Read the model definition and answer for the solid it produces. Units are mm, in the model's axes. A direction names the side the tool comes from. Coordinates: 2 decimals unless noted, no trailing zeros. Loops run counter-clockwise (first coordinate to the right, second up) from the corner with the lowest first, then second, coordinate; pieces in that order, holes last.
from build123d import *

# Parameters (mm, degrees)
SKETCH_1_W          = 21
SKETCH_1_H          = 31
EXTRUDE_1_DEPTH     = 20
CUT_EXTRUDE_5_REACH = 50.177
SKETCH_14_R         = 1.5
CUT_EXTRUDE_6_REACH = 50.177
SKETCH_15_R         = 1.5
EXTRUDE_2_DEPTH     = 1
EXTRUDE_START       = 1
EXTRUDE_3_DEPTH     = 1
SKETCH_4_R          = 1.5
CUT_EXTRUDE_1_DEPTH = 3
SKETCH_5_R          = 5
CUT_EXTRUDE_2_DEPTH = 4
SKETCH_6_W          = 9
SKETCH_6_H          = 29
EXTRUDE_START_2     = -8
SKETCH_7_R          = 1.5
EXTRUDE_4_DEPTH     = 8
EXTRUDE_START_3     = 20
SKETCH_8_R          = 5
EXTRUDE_5_DEPTH     = 20
SKETCH_10_R         = 1.75
CUT_EXTRUDE_4_DEPTH = 20
SKETCH_9_R          = 5
SKETCH_9_R_2        = 4
CUT_EXTRUDE_3_DEPTH = 1
SKETCH_11_R         = 2.85
EXTRUDE_6_DEPTH     = 3.5
FILLET_1_R          = 0.5
CHAMFER_1_SIZE      = 0.5


with BuildPart() as part:
    # ｽｹｯﾁ1 → ﾎﾞｽ - 押し出し1 (new body)
    with BuildSketch(Plane(origin=(0, 0, 0), x_dir=(1, 0, 0), z_dir=(0, 1, 0))):
        with BuildLine():
            Line((2, 0), (23, 0))
            ThreePointArc((23, 0), (24.414213562, 0.585786438), (25, 2))
            Line((25, 2), (25, 36))
            Line((25, 36), (0, 36))
            Line((0, 36), (0, 2))
            ThreePointArc((0, 2), (0.585786438, 0.585786438), (2, 0))
        make_face()
        with Locations((12.5, 17.5)):
            Rectangle(SKETCH_1_W, SKETCH_1_H, mode=Mode.SUBTRACT)
    extrude(amount=EXTRUDE_1_DEPTH)

    # ｽｹｯﾁ14 → ｶｯﾄ - 押し出し5 (cut, up to next)
    with BuildSketch(Plane(origin=(25, 0, 0), x_dir=(0, 0, -1), z_dir=(1, 0, 0)), mode=Mode.PRIVATE) as cut_extrude_5_sk1:
        with Locations((9, 6)):
            Circle(SKETCH_14_R)
    cut_extrude_5_tool1 = extrude(cut_extrude_5_sk1.sketch, amount=-CUT_EXTRUDE_5_REACH, mode=Mode.PRIVATE) & part.part
    # ｽｹｯﾁ14 → ｶｯﾄ - 押し出し5 (cut, up to next)
    with BuildSketch(Plane(origin=(25, 0, 0), x_dir=(0, 0, -1), z_dir=(1, 0, 0)), mode=Mode.PRIVATE) as cut_extrude_5_sk2:
        with Locations((28, 14)):
            Circle(SKETCH_14_R)
    cut_extrude_5_tool2 = extrude(cut_extrude_5_sk2.sketch, amount=-CUT_EXTRUDE_5_REACH, mode=Mode.PRIVATE) & part.part
    add(cut_extrude_5_tool1.solids().sort_by_distance((25, 6, -9))[0], mode=Mode.SUBTRACT)
    add(cut_extrude_5_tool2.solids().sort_by_distance((25, 14, -28))[0], mode=Mode.SUBTRACT)

    # ｽｹｯﾁ15 → ｶｯﾄ - 押し出し6 (cut, up to next)
    with BuildSketch(Plane.ZY, mode=Mode.PRIVATE) as cut_extrude_6_sk1:
        with Locations((-28, 6)):
            Circle(SKETCH_15_R)
    cut_extrude_6_tool1 = extrude(cut_extrude_6_sk1.sketch, amount=-CUT_EXTRUDE_6_REACH, mode=Mode.PRIVATE) & part.part
    # ｽｹｯﾁ15 → ｶｯﾄ - 押し出し6 (cut, up to next)
    with BuildSketch(Plane.ZY, mode=Mode.PRIVATE) as cut_extrude_6_sk2:
        with Locations((-9, 14)):
            Circle(SKETCH_15_R)
    cut_extrude_6_tool2 = extrude(cut_extrude_6_sk2.sketch, amount=-CUT_EXTRUDE_6_REACH, mode=Mode.PRIVATE) & part.part
    add(cut_extrude_6_tool1.solids().sort_by_distance((0, 6, -28))[0], mode=Mode.SUBTRACT)
    add(cut_extrude_6_tool2.solids().sort_by_distance((0, 14, -9))[0], mode=Mode.SUBTRACT)

    # ｽｹｯﾁ2 → ﾎﾞｽ - 押し出し2 (add)
    with BuildSketch(Plane(origin=(0, 0, -2), x_dir=(-1, 0, 0), z_dir=(0, 0, -1))):
        with BuildLine():
            Line((-22.4, 0.1), (-2.6, 0.1))
            ThreePointArc((-2.6, 0.1), (-2.246446609, 0.246446609), (-2.1, 0.6))
            Line((-2.1, 0.6), (-2.1, 19.4))
            ThreePointArc((-2.1, 19.4), (-2.246446609, 19.753553391), (-2.6, 19.9))
            Line((-2.6, 19.9), (-22.4, 19.9))
            ThreePointArc((-22.4, 19.9), (-22.753553391, 19.753553391), (-22.9, 19.4))
            Line((-22.9, 19.4), (-22.9, 0.6))
            ThreePointArc((-22.9, 0.6), (-22.753553391, 0.246446609), (-22.4, 0.1))
        make_face()
    extrude(amount=EXTRUDE_2_DEPTH)

    # ｽｹｯﾁ3 → ﾎﾞｽ - 押し出し3 (add)
    with BuildSketch(Plane.XY.offset(-33).offset(EXTRUDE_START)):
        with BuildLine():
            Line((2.6, 0.1), (22.4, 0.1))
            ThreePointArc((22.4, 0.1), (22.753553391, 0.246446609), (22.9, 0.6))
            Line((22.9, 0.6), (22.9, 19.4))
            ThreePointArc((22.9, 19.4), (22.753553391, 19.753553391), (22.4, 19.9))
            Line((22.4, 19.9), (2.6, 19.9))
            ThreePointArc((2.6, 19.9), (2.246446609, 19.753553391), (2.1, 19.4))
            Line((2.1, 19.4), (2.1, 0.6))
            ThreePointArc((2.1, 0.6), (2.246446609, 0.246446609), (2.6, 0.1))
        make_face()
    extrude(amount=-EXTRUDE_3_DEPTH)

    # ｽｹｯﾁ4 → ｶｯﾄ - 押し出し1 (cut)
    with BuildSketch(Plane.XY):
        with Locations((12.5, 10)):
            Circle(SKETCH_4_R)
    extrude(amount=-CUT_EXTRUDE_1_DEPTH, mode=Mode.SUBTRACT)

    # ｽｹｯﾁ5 → ｶｯﾄ - 押し出し2 (cut)
    with BuildSketch(Plane(origin=(0, 0, -36), x_dir=(-1, 0, 0), z_dir=(0, 0, -1))):
        with Locations((-12.5, 10)):
            Circle(SKETCH_5_R)
    extrude(amount=-CUT_EXTRUDE_2_DEPTH, mode=Mode.SUBTRACT)

    # ｽｹｯﾁ6 → 回転1 (revolve)
    with BuildSketch(Plane(origin=(0, 10, 0), x_dir=(1, 0, 0), z_dir=(0, 1, 0))):
        with Locations((8, 17.5)):
            Rectangle(SKETCH_6_W, SKETCH_6_H)
    revolve(axis=Axis((12.5, 10, -32), (0, 0, 1)))

    # ｽｹｯﾁ7 → ﾎﾞｽ - 押し出し4 (add)
    with BuildSketch(Plane(origin=(0, 0, -3), x_dir=(-1, 0, 0), z_dir=(0, 0, -1)).offset(EXTRUDE_START_2)):
        with Locations((-12.5, 10)):
            Circle(SKETCH_7_R)
    extrude(amount=EXTRUDE_4_DEPTH)

    # ｽｹｯﾁ8 → ﾎﾞｽ - 押し出し5 (add)
    with BuildSketch(Plane(origin=(0, 0, -32), x_dir=(-1, 0, 0), z_dir=(0, 0, -1)).offset(EXTRUDE_START_3)):
        with Locations((-12.5, 10)):
            Circle(SKETCH_8_R)
    extrude(amount=-EXTRUDE_5_DEPTH)

    # ｽｹｯﾁ10 → ｶｯﾄ - 押し出し4 (cut)
    with BuildSketch(Plane(origin=(0, 0, -52), x_dir=(-1, 0, 0), z_dir=(0, 0, -1))):
        with Locations((-12.5, 10)):
            Circle(SKETCH_10_R)
    extrude(amount=-CUT_EXTRUDE_4_DEPTH, mode=Mode.SUBTRACT)

    # ｽｹｯﾁ9 → ｶｯﾄ - 押し出し3 (cut)
    with BuildSketch(Plane(origin=(0, 0, -50), x_dir=(-1, 0, 0), z_dir=(0, 0, -1))):
        with Locations((-12.5, 10)):
            Circle(SKETCH_9_R)
        with Locations((-12.5, 10)):
            Circle(SKETCH_9_R_2, mode=Mode.SUBTRACT)
    extrude(amount=-CUT_EXTRUDE_3_DEPTH, mode=Mode.SUBTRACT)

    # ｽｹｯﾁ11 → ﾎﾞｽ - 押し出し6 (add)
    with BuildSketch(Plane.XY.offset(6)):
        with Locations((12.5, 10)):
            Circle(SKETCH_11_R)
    extrude(amount=-EXTRUDE_6_DEPTH)

    # ｽｹｯﾁ12 → 回転2 (revolve)
    with BuildSketch(Plane.ZY.offset(-12.5), mode=Mode.PRIVATE) as revolve_2_sk:
        with BuildLine():
            Line((6, 10), (7, 10))
            ThreePointArc((7, 10), (6.742745419, 11.510173831), (6, 12.85))
            Line((6, 12.85), (6, 10))
        make_face()
    revolve(revolve_2_sk.sketch.rotate(Axis((12.5, 10, 6), (0, 0, 1)), 270), axis=Axis((12.5, 10, 6), (0, 0, 1)))

    # ﾌｨﾚｯﾄ1
    fillet_1_edges = [part.edges().sort_by_distance(p)[0] for p in [
        (9.65, 10, 6),
    ]]
    fillet(fillet_1_edges, radius=FILLET_1_R)

    # 面取り1
    chamfer_1_edges = [part.edges().sort_by_distance(p)[0] for p in [
        (17.5, 10, -52),
    ]]
    chamfer(chamfer_1_edges, length=CHAMFER_1_SIZE)


solid = part.part
Q1. Flat-ended cylindrical pins translate along their axes: pin 1 Ø6 at (x, y) = (4, 10.5) entering from -Z; pin 2 Ø2.5 at (y, z) = (6, -9) entering from +X; pin 3 Ø1 at (x, z) = (17.5, -3) entering from -Y. Find the tip coordinate at first contact, or state that the pin passes through.
Findings below:
pin 1: stops at z = -36
pin 2: stops at x = 21.07
pin 3: stops at y = 0.1
Q2. Which of the six approach directions +Z, -Z, +X, -X, +Y, -Y give full straight-line access (tool end or side, diameter ignored) to faces 1 (the face through (0.99, 14.07, -10.5)), 2 (the face through (23, 10, -17)), 3 (the face through (14, 9, 2.5)), 4 (the face through (24.01, 14.07, -26.5)), 5 (the face through (13, 10, -32))?
Findings below:
face 1: -X
face 2: +Y, -Y
face 3: none
face 4: +X
face 5: -Z
Q3. A cutting plane is placed at A-A (z = -31). Give the vertices of the cut face in (x, y), then the cut area to 3 significant figures.
Findings below:
outline: (0, 0) - (2, 0) - (2, 20) - (0, 20) - close; circle Ø18 at (12.5, 10); (23, 0) - (25, 0) - (25, 20) - (23, 20) - close
area: 334 mm2
Q4. Determine the mould class of faces 6 (the face through (14.451, 18.786, -17.703)), 7 (the face through (12, 12, 0)), 8 (the face through (24, 5.1, -7.8)) for opening direction Y: +Y half, -Y half, draft (parallel to the pull), parting line (faces both ways), or undercut.
Findings below:
face 6: parting line
face 7: draft
face 8: undercut
Q5. A cutting plane is placed at D-D (x = 20.25). Give the vertices of the cut face in (y, z), then the cut area to 3 significant figures.
Findings below:
outline: (0, -36) - (20, -36) - (20, -33) - (19.9, -33) - (19.9, -32) - (14.58, -32) - (14.58, -3) - (19.9, -3) - (19.9, -2) - (20, -2) - (20, 0) - (0, 0) - (0, -2) - (0.1, -2) - (0.1, -3) - (5.42, -3) - (5.42, -32) - (0.1, -32) - (0.1, -33) - (0, -33) - close
area: 405 mm2
Q6. Straight lines are drawn through the part: probe 1 along Z at (x, y) = (2.75, 8); probe 2 along X at (y, z) = (2.25, -19); probe 3 along Y at (x, z) = (12.5, -43.5). For each, find the intervals that lie inside material, in ascending order.
Findings below:
probe 1: z = -36 to -32, -3 to 0
probe 2: x = 0 to 2, 7.92 to 17.08, 23 to 25
probe 3: y = 5 to 8.25, 11.75 to 15
Q7. A cutting plane is placed at C-C (z = -47.5). Give the vertices of the cut face in (x, y).
Findings below:
outline: circle Ø10 at (12.5, 10); hole circle Ø3.5 at (12.5, 10)
Q8. A cutting plane is placed at B-B (z = -9). Give the vertices of the cut face in (x, y), then the cut area to 3 significant figures.
Findings below:
outline: (0, 0) - (2, 0) - (2, 12.5) - (0, 12.5) - close; (0, 15.5) - (2, 15.5) - (2, 20) - (0, 20) - close; circle Ø18 at (12.5, 10); (23, 0) - (25, 0) - (25, 4.5) - (23, 4.5) - close; (23, 7.5) - (25, 7.5) - (25, 20) - (23, 20) - close
area: 322 mm2
